For this review, take the finished solid that the model builds, in its own axes (mm). A direction names the side the tool comes from. Give positions to 0.01 mm unless a question says otherwise; leave off trailing zeros. Write each loop counter-clockwise with the first axis right and the second up, starting at its lowest first coordinate (ties: lowest second). Pieces come first, ordered by that corner, then holes. Notation, with made-up numbers: (84, 69.5) -> (114, 69.5) arc R9 cw to (114, 76.5) -> close; hole circle Ø8 at (38.5, 3). An arc over 180 degrees is marked (long way). Answer as CSV lines item,"result".
```python
from build123d import *

# Parameters (mm, degrees)
SKETCH2_W           = 128
SKETCH2_H           = 86
BOSS_EXTRUDE1_DEPTH = 2.5
SKETCH9_W           = 8.5
SKETCH9_H           = 2
BOSS_EXTRUDE3_DEPTH = 6.5
CUT_EXTRUDE9_START  = 3.5
SKETCH10_W          = 8.5
SKETCH10_H          = 2
CUT_EXTRUDE9_DEPTH  = 74.877322259
FILLET1_R           = 0.5
SKETCH3_W           = 25
SKETCH3_H           = 35
CUT_EXTRUDE10_DEPTH = 1.5
SKETCH11_W          = 17
SKETCH11_H          = 26
CUT_EXTRUDE11_DEPTH = 10
SKETCH12_W          = 7
SKETCH12_H          = 75
SKETCH12_W_2        = 4
SKETCH12_H_2        = 20
BOSS_EXTRUDE4_DEPTH = 2.5


with BuildPart() as part:
    # Sketch2 → Boss-Extrude1 (new body)
    with BuildSketch(Plane(origin=(0, 0, 0), x_dir=(1, 0, 0), z_dir=(0, 1, 0))):
        Rectangle(SKETCH2_W, SKETCH2_H)
    extrude(amount=-BOSS_EXTRUDE1_DEPTH)

    # Sketch9 → Boss-Extrude3 (add)
    with BuildSketch(Plane(origin=(0, 0, 0), x_dir=(1, 0, 0), z_dir=(0, 1, 0))):
        Polygon((-61.5, -20), (-60.5, -20), (-60.5, 39), (-40.5, 39), (-40.5, 40), (-61.5, 40), align=None)
        Polygon((40.5, 40), (61.5, 40), (61.5, -20), (60.5, -20), (60.5, 39), (40.5, 39), align=None)
        with Locations((-5, 40)):
            Rectangle(SKETCH9_W, SKETCH9_H)
        with Locations((5, 40)):
            Rectangle(SKETCH9_W, SKETCH9_H)
        with Locations((-5, -40)):
            Rectangle(SKETCH9_W, SKETCH9_H)
        with Locations((5, -40)):
            Rectangle(SKETCH9_W, SKETCH9_H)
    extrude(amount=BOSS_EXTRUDE3_DEPTH)

    # Sketch10 → Cut-Extrude9 (cut, through all)
    with BuildSketch(Plane(origin=(0, 0, 0), x_dir=(1, 0, 0), z_dir=(0, 1, 0)).offset(CUT_EXTRUDE9_START)):
        with Locations((-5, 40)):
            Rectangle(SKETCH10_W, SKETCH10_H)
        with Locations((5, 40)):
            Rectangle(SKETCH10_W, SKETCH10_H)
        with Locations((-5, -40)):
            Rectangle(SKETCH10_W, SKETCH10_H)
        with Locations((5, -40)):
            Rectangle(SKETCH10_W, SKETCH10_H)
    extrude(amount=CUT_EXTRUDE9_DEPTH, mode=Mode.SUBTRACT)

    # Fillet1
    fillet1_edges = [part.edges().sort_by_distance(p)[0] for p in [
        (0.75, 3.5, -40),
        (9.25, 3.5, -40),
        (-9.25, 3.5, 40),
        (-0.75, 3.5, 40),
        (0.75, 3.5, 40),
        (9.25, 3.5, 40),
        (-9.25, 3.5, -40),
        (-0.75, 3.5, -40),
        (40.5, 6.5, -39.5),
        (61, 6.5, 20),
        (-61, 6.5, 20),
        (-40.5, 6.5, -39.5),
    ]]
    fillet(fillet1_edges, radius=FILLET1_R)

    # Sketch3 → Cut-Extrude10 (cut)
    with BuildSketch(Plane(origin=(0, 0, 0), x_dir=(1, 0, 0), z_dir=(0, 1, 0))):
        with Locations((-35, 20)):
            Rectangle(SKETCH3_W, SKETCH3_H)
        with Locations((-35, -20)):
            Rectangle(SKETCH3_W, SKETCH3_H)
        with Locations((0, 20)):
            Rectangle(SKETCH3_W, SKETCH3_H)
        with Locations((0, -20)):
            Rectangle(SKETCH3_W, SKETCH3_H)
        with Locations((35, 20)):
            Rectangle(SKETCH3_W, SKETCH3_H)
        with Locations((35, -20)):
            Rectangle(SKETCH3_W, SKETCH3_H)
    extrude(amount=-CUT_EXTRUDE10_DEPTH, mode=Mode.SUBTRACT)

    # Sketch11 → Cut-Extrude11 (cut)
    with BuildSketch(Plane(origin=(0, 0, 0), x_dir=(1, 0, 0), z_dir=(0, 1, 0))):
        with Locations((0, -20)):
            Rectangle(SKETCH11_W, SKETCH11_H)
        with Locations((-35, -20)):
            Rectangle(SKETCH11_W, SKETCH11_H)
        with Locations((0, 20)):
            Rectangle(SKETCH11_W, SKETCH11_H)
        with Locations((35, 20)):
            Rectangle(SKETCH11_W, SKETCH11_H)
        with Locations((35, -20)):
            Rectangle(SKETCH11_W, SKETCH11_H)
        with Locations((-35, 20)):
            Rectangle(SKETCH11_W, SKETCH11_H)
    extrude(amount=-CUT_EXTRUDE11_DEPTH, mode=Mode.SUBTRACT)

    # Sketch12 → Boss-Extrude4 (add)
    # profile 1 of 4: a face of its own
    with BuildSketch(Plane(origin=(0, 0, 0), x_dir=(1, 0, 0), z_dir=(0, 1, 0))):
        with Locations((-17.5, 0)):
            Rectangle(SKETCH12_W, SKETCH12_H)
        with Locations((-17.5, 0)):
            Rectangle(SKETCH12_W_2, SKETCH12_H_2, mode=Mode.SUBTRACT)
        with Locations((-17.5, 25)):
            Rectangle(SKETCH12_W_2, SKETCH12_H_2, mode=Mode.SUBTRACT)
        with Locations((-17.5, -25)):
            Rectangle(SKETCH12_W_2, SKETCH12_H_2, mode=Mode.SUBTRACT)
    # profile 2 of 4: a face of its own
    with BuildSketch(Plane(origin=(0, 0, 0), x_dir=(1, 0, 0), z_dir=(0, 1, 0))):
        with Locations((-52.5, 0)):
            Rectangle(SKETCH12_W, SKETCH12_H)
        with Locations((-52.5, -25)):
            Rectangle(SKETCH12_W_2, SKETCH12_H_2, mode=Mode.SUBTRACT)
        with Locations((-52.5, 0)):
            Rectangle(SKETCH12_W_2, SKETCH12_H_2, mode=Mode.SUBTRACT)
        with Locations((-52.5, 25)):
            Rectangle(SKETCH12_W_2, SKETCH12_H_2, mode=Mode.SUBTRACT)
    # profile 3 of 4: a face of its own
    with BuildSketch(Plane(origin=(0, 0, 0), x_dir=(1, 0, 0), z_dir=(0, 1, 0))):
        with Locations((17.5, 0)):
            Rectangle(SKETCH12_W, SKETCH12_H)
        with Locations((17.5, -25)):
            Rectangle(SKETCH12_W_2, SKETCH12_H_2, mode=Mode.SUBTRACT)
        with Locations((17.5, 0)):
            Rectangle(SKETCH12_W_2, SKETCH12_H_2, mode=Mode.SUBTRACT)
        with Locations((17.5, 25)):
            Rectangle(SKETCH12_W_2, SKETCH12_H_2, mode=Mode.SUBTRACT)
    # profile 4 of 4: a face of its own
    with BuildSketch(Plane(origin=(0, 0, 0), x_dir=(1, 0, 0), z_dir=(0, 1, 0))):
        with Locations((52.5, 0)):
            Rectangle(SKETCH12_W, SKETCH12_H)
        with Locations((52.5, -25)):
            Rectangle(SKETCH12_W_2, SKETCH12_H_2, mode=Mode.SUBTRACT)
        with Locations((52.5, 0)):
            Rectangle(SKETCH12_W_2, SKETCH12_H_2, mode=Mode.SUBTRACT)
        with Locations((52.5, 25)):
            Rectangle(SKETCH12_W_2, SKETCH12_H_2, mode=Mode.SUBTRACT)
    extrude(amount=BOSS_EXTRUDE4_DEPTH)


solid = part.part
```
Q1. Add section D-D (z = 29). State how many separate pieces and enclosed holes the cut face has, plus the area to 4 significant figures.
Answer block:
separate pieces,"4"
enclosed holes,"0"
area,"186.5 mm2"
Q2. Clearance check with flat-ended pins moving along their axes: pin 1 (2 mm diameter, centred on x = 4, z = -40.5, fed in from +Y); pin 2 (3 mm diameter, centred on x = 52.5, z = -4.5, fed in from +Y); pin 3 (3 mm diameter, centred on y = 1, z = -1.5, fed in from +X); pin 4 (5 mm diameter, centred on y = 3, z = -3, fed in from -X). State where each tip first meets the part, or that it passes through.
Answer block:
pin 1,"stops at y = 3.5"
pin 2,"stops at y = 0"
pin 3,"stops at x = 64"
pin 4,"stops at x = -61.5"
Q3. Draft analysis for pull direction Z (two halves, no side actions). For faces 6 (the flat face through (-53, 1, 35)), 7 (the flat face through (-50.5, 1, 25)), 8 (the flat face through (-53, 1, 37.5)), 9 (the flat face through (-51, 3, -40)), state which applies: released by +Z, released by -Z, zero draft, split by the parting line, or undercut.
Answer block:
face 6,"undercut"
face 7,"undercut"
face 8,"released by +Z"
face 9,"released by -Z"
Q4. For faces 1 (the flat face through (5, 2, 39)), 2 (the flat face through (51, 3, -40)), 3 (the flat face through (-18, 1, 37.5)), 4 (the flat face through (-18, 1, -35)), 5 (the flat face through (-55, 2.5, -1)), list the 3-axis set-ups (+Z, -Z, +X, -X, +Y, -Y) from which the entire face can be reached by the end or side of a thin tool; tool diameter is ignored.
Answer block:
face 1,"+X, -X, +Y"
face 2,"-Z, +X, +Y"
face 3,"+Z, +X, -X, +Y"
face 4,"+Y"
face 5,"+Z, +Y"
Q5. To check wall thickness, follow probe 1 along X at (y, z) = (-0.25, 35); probe 2 along Z at (x, y) = (-36.5, -1); probe 3 along X at (y, z) = (5.5, 17.5). State the ranges of each line that lie inside material, in increasing order. Write a range as [from, to].
Answer block:
probe 1,"x = [-64, -47.5], [-22.5, -12.5], [12.5, 22.5], [47.5, 64]"
probe 2,"z = [-43, -37.5], [-2.5, 2.5], [37.5, 43]"
probe 3,"x = [-61.5, -60.5], [60.5, 61.5]"
Q6. Add section A-A (x = -30). Write out the cut boundary in (y, z).
Answer block:
outline,"(-2.5, -43) -> (0, -43) -> (0, -37.5) -> (-1.5, -37.5) -> (-1.5, -33) -> (-2.5, -33) -> close; (-2.5, -7) -> (-1.5, -7) -> (-1.5, -2.5) -> (0, -2.5) -> (0, 2.5) -> (-1.5, 2.5) -> (-1.5, 7) -> (-2.5, 7) -> close; (-2.5, 33) -> (-1.5, 33) -> (-1.5, 37.5) -> (0, 37.5) -> (0, 43) -> (-2.5, 43) -> close"
Q7. Add section B-B (y = 4.75). Write out the cut boundary in (x, z), plus the area to 3 significant figures.
Answer block:
outline,"(-61.5, -40) -> (-40.5, -40) -> (-40.5, -39) -> (-60.5, -39) -> (-60.5, 20) -> (-61.5, 20) -> close; (40.5, -40) -> (61.5, -40) -> (61.5, 20) -> (60.5, 20) -> (60.5, -39) -> (40.5, -39) -> close"
area,"160 mm2"
Q8. Add section C-C (x = 46). Write out the cut boundary in (y, z), plus the area to 4 significant figures.
Answer block:
outline,"(-2.5, -43) -> (0, -43) -> (0, -40) -> (6.5, -40) -> (6.5, -39) -> (0, -39) -> (0, -37.5) -> (-1.5, -37.5) -> (-1.5, -2.5) -> (0, -2.5) -> (0, 2.5) -> (-1.5, 2.5) -> (-1.5, 37.5) -> (0, 37.5) -> (0, 43) -> (-2.5, 43) -> close"
area,"116.5 mm2"
